The model under review builds one solid part; all positions refer to its coordinate system, in mm. Round coordinates to 2 decimals unless told otherwise and drop trailing zeros. Loops run counter-clockwise (first coordinate to the right, second up) from the corner with the lowest first, then second, coordinate; pieces in that order, holes last. Notation, with made-up numbers: M 89.5,68 L 96.5,68 A20 ccw 96.5,98 Z; hole C -26,14 d8. An arc over 180 degrees is marked long. Return JSON: item names as keys, results as strings. Group by question number.
Q1. Consider section B-B (x = 68.5). State the section outline as (y, z) points, and give its area (3 significant figures).
Q2. To check wall thickness, follow line 1 along Y through (x, z) = (98, 0.3); line 2 along Y through (x, z) = (117.5, 0.2); line 3 along Z through (x, y) = (82, 5.5). State the ranges of each line that lie inside material, in increasing order.
Q3. Draft analysis for pull direction Y (two halves, no side actions). For faces 1 (the face through (80, 11.112, 1)), 2 (the face through (78, 6, 0.254)), 3 (the face through (78, 0, 1)), state which applies: pulls with the +Y half, pulls with the -Y half, needs draft (parallel to the pull), parting line crosses it, or undercut.
Q4. Clearance check with a flat-ended pin moving along its axis: pin 1 Ø2.5 at (x, y) = (62, 5) entering from +Z. State where the tip first meets the part, or that it passes through.
Q5. Consider section A-A (z = 1.8). State the section outline as (x, y) points.
Q6. Consider section C-C (y = 8). State the section outline as (x, z) points.
Autodesk Inventor part; units mm, degrees
ref_plane "YZ Plane" through (0, 0, 0) normal (1, 0, 0) x (0, 1, 0)
ref_plane "XZ Plane" through (0, 0, 0) normal (0, 1, 0) x (-1, 0, 0)
ref_plane "XY Plane" through (0, 0, 0) normal (0, 0, 1) x (1, 0, 0)
sketch "Sketch1" plane through (0, 0, 0) normal (0, 0, 1) x (1, 0, 0)
  line L0 (0, 0) -> (157.48, 0)
  line L1 (157.48, 0) -> (157.48, 11.1125)
  line L2 (157.48, 11.1125) -> (0, 11.1125)
  line L3 (0, 11.1125) -> (0, 0)
  line L4 (0, 11.1125) -> (157.48, 11.1125)
  line L5 (157.48, 11.1125) -> (157.48, 9.8425)
  line L6 (157.48, 9.8425) -> (0, 9.8425)
  line L7 (0, 9.8425) -> (0, 11.1125)
  line L8 (0, 0) -> (157.48, 0)
  line L9 (157.48, 0) -> (157.48, 1.27)
  line L10 (157.48, 1.27) -> (0, 1.27)
  line L11 (0, 1.27) -> (0, 0)
  line L12 (11.0159, 5.08) -> (19.9525, 5.08)
  line L13 (19.9525, 5.08) -> (19.9525, 6.0325)
  line L14 (19.9525, 6.0325) -> (11.0159, 6.0325)
  line L15 (11.0159, 6.0325) -> (11.0159, 5.08)
  line L16 (70.7525, 5.08) -> (70.7525, 6.0325)
  line L17 (70.7525, 6.0325) -> (61.8159, 6.0325)
  line L18 (61.8159, 5.08) -> (70.7525, 5.08)
  line L19 (61.8159, 6.0325) -> (61.8159, 5.08)
  line L20 (121.5525, 5.08) -> (121.5525, 6.0325)
  line L21 (121.5525, 6.0325) -> (112.6159, 6.0325)
  line L22 (112.6159, 5.08) -> (121.5525, 5.08)
  line L23 (112.6159, 6.0325) -> (112.6159, 5.08)
  point P0 (39.5656, 5.08)
  point P1 (47.7905, 6.0325)
  point P2 (98.5905, 6.0325)
  point P3 (90.3656, 5.08)
  point P4 (149.3905, 6.0325)
  point P5 (141.1656, 5.08)
  point P6 (0, 9.8425)
  point P7 (0, 1.27)
  dimension "d0" = 157.48
  dimension "d1" = 11.1125
  dimension "d2" = 1.27
  dimension "d3" = 1.27
  dimension "d4" = 3.81
  dimension "d5" = 3.81
  dimension "d6" = 8.9366
  dimension "d9" = 50.8
extrude "Extrusion1" add sketch "Sketch1" along normal blind 2.54 contours L3 L10 L1 L0 | L3 L2 L1 L6
extrude "Extrusion2" add sketch "Sketch1" along normal blind 0.254 contours L3 L6 L1 L10
properties part number "Bracket holder"
Values:
{
 "1": {"outline": "M 0,0 L 5.08,0 L 5.08,0.25 L 1.27,0.25 L 1.27,2.54 L 0,2.54 Z; M 6.03,0 L 11.11,0 L 11.11,2.54 L 9.84,2.54 L 9.84,0.25 L 6.03,0.25 Z", "area": "8.39 mm2"},
 "2": {"line 1": "y = 0 to 1.27, 9.84 to 11.11", "line 2": "y = 0 to 5.08, 6.03 to 11.11", "line 3": "z = 0 to 0.25"},
 "3": {"face 1": "pulls with the +Y half", "face 2": "undercut", "face 3": "pulls with the -Y half"},
 "4": {"pin 1": "stops at z = 0.25"},
 "5": {"outline": "M 0,0 L 157.48,0 L 157.48,1.27 L 0,1.27 Z; M 0,9.84 L 157.48,9.84 L 157.48,11.11 L 0,11.11 Z"},
 "6": {"outline": "M 0,0 L 157.48,0 L 157.48,0.25 L 0,0.25 Z"}
}
